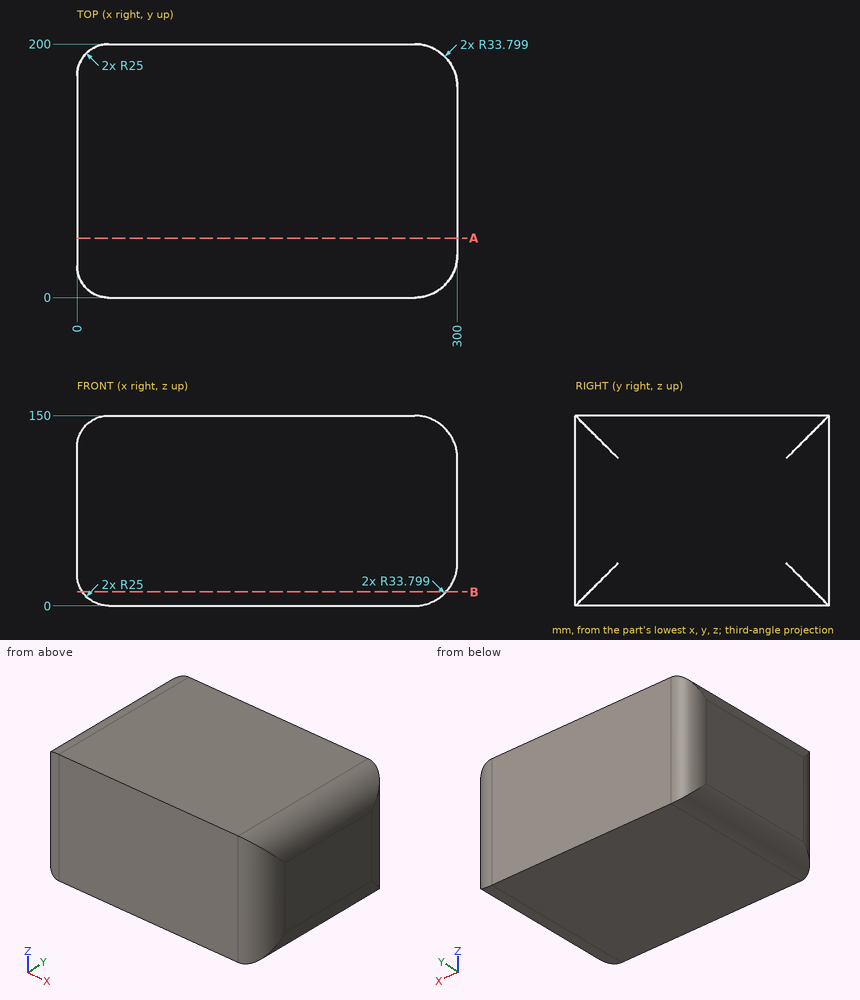
Geometry check sheet. Reference: drawing and pictorial views, mm from the part's lowest x, y, z. Coordinates: 2 decimals unless noted, no trailing zeros. Order: outer loops, then holes, each group sorted by start corner. A loop starts at its lowest first (then second) coordinate and runs counter-clockwise, first axis right, second up.
1. Go/stop test with a flat-tipped pin: pin 1 Ø3 at (y, z) = (50.5, 19.5) entering from -X. Record where the tip stops, or that it passes through.
Results found:
pin 1: stops at x = 0.32
2. Sectioned sample at A-A, the plane y = 47. Record the cut outline in (x, z), and give its area (3 significant figures).
Results found:
outline: (0, 25) arc R25 ccw to (25, 0) - (266.2, 0) arc R33.8 ccw to (300, 33.8) - (300, 116.2) arc R33.8 ccw to (266.2, 150) - (25, 150) arc R25 ccw to (0, 125) - close
area: 44,200 mm2
3. Sectioned sample at B-B, the plane z = 11. Record the cut outline in (x, y).
Results found:
outline: (4.29, 11) arc R25 ccw to (25, 0) - (266.2, 0) arc R33.8 ccw to (291.15, 11) - (291.15, 189) arc R33.8 ccw to (266.2, 200) - (25, 200) arc R25 ccw to (4.29, 189) - close
4. Scan lines: line 1 (Z direction, x = 268, y = 85.5); line 2 (Y direction, x = 285.5, z = 53.5); line 3 (X direction, y = 180, z = 117). Record each from-to range of solid material in increasing order.
Results found:
line 1: z = 0.05 to 149.95
line 2: y = 6.05 to 193.95
line 3: x = 0.51 to 297.05
